Drawing for the job (mm, zero at the part's lowest x, y, z). A direction names the side the tool comes from. Round coordinates to 2 decimals unless told otherwise and drop trailing zeros. Loops run counter-clockwise (first coordinate to the right, second up) from the corner with the lowest first, then second, coordinate; pieces in that order, holes last. Notation, with made-up numbers: M 13.25,49.25 L 69.25,49.25 A16 ccw 69.25,71.25 Z; hole C 51,-3.75 d5. An arc over 180 degrees is marked long. Answer in a Markdown table with one row per item.
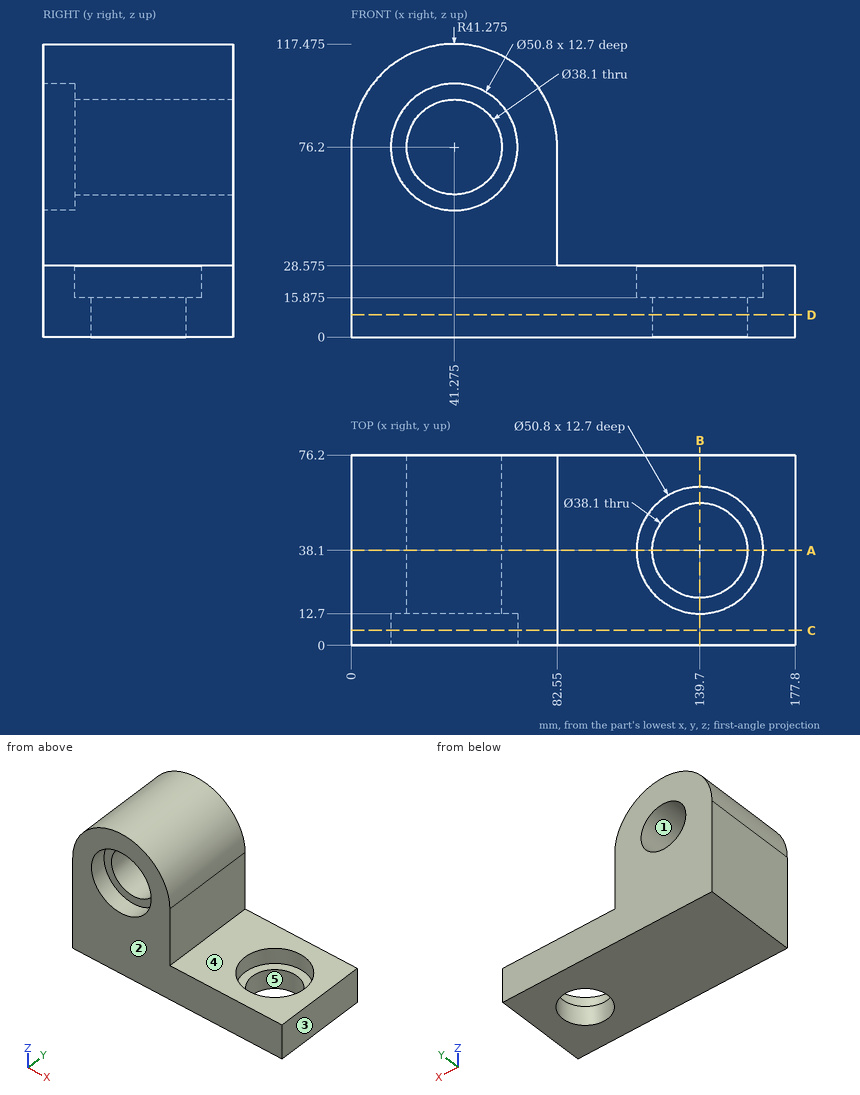
1. Saw through at A-A (y = 38.1). Write the cut outline in (x, z) (3 decimals), and give its area (3 significant figures).
Verdict:
| item | result |
|---|---|
| outline | M 0,0 L 120.65,0 L 120.65,15.875 L 114.3,15.875 L 114.3,28.575 L 82.55,28.575 L 82.55,76.2 A41.275 ccw 0,76.2 Z; M 158.75,0 L 177.8,0 L 177.8,28.575 L 165.1,28.575 L 165.1,15.875 L 158.75,15.875 Z; hole C 41.275,76.2 d38.1 |
| area | 9,300 mm² |
2. Saw through at B-B (x = 139.7). Write the cut outline in (y, z) (3 decimals).
Verdict:
| item | result |
|---|---|
| outline | M 0,0 L 19.05,0 L 19.05,15.875 L 12.7,15.875 L 12.7,28.575 L 0,28.575 Z; M 57.15,0 L 76.2,0 L 76.2,28.575 L 63.5,28.575 L 63.5,15.875 L 57.15,15.875 Z |
3. Saw through at D-D (z = 9). Write the cut outline in (x, y), and give its area (3 significant figures).
Verdict:
| item | result |
|---|---|
| outline | M 0,0 L 177.8,0 L 177.8,76.2 L 0,76.2 Z; hole C 139.7,38.1 d38.1 |
| area | 12,400 mm² |
4. Tool access for the marked faces 4 and 5: list every direction of +Z, -Z, +X, -X, +Y, -Y with a clear straight run to the whole face (end or side of a thin tool).
Verdict:
| item | result |
|---|---|
| face 4 | +Z, +X, +Y, -Y |
| face 5 | +Z, -Z |
5. Pin check, flat tips, straight feed: pin 1 (6 mm diameter, centred on y = 25, z = 71.5, fed in from +X); pin 2 (4 mm diameter, centred on x = 65, y = 10.5, fed in from +Z); pin 3 (6 mm diameter, centred on y = 56.5, z = 98.5, fed in from +X). Stop position of each tip, or through.
Verdict:
| item | result |
|---|---|
| pin 1 | stops at x = 82.55 |
| pin 2 | stops at z = 111.29 |
| pin 3 | stops at x = 77.76 |
6. Mould opens along X. For the marked faces 1, 2 and 3 say: +X half, -X half, draft (parallel to the pull), parting line (faces both ways), or undercut.
Verdict:
| item | result |
|---|---|
| face 1 | undercut |
| face 2 | draft |
| face 3 | +X half |
7. Saw through at C-C (y = 6). Write the cut outline in (x, z) (3 decimals), and give its area (3 significant figures).
Verdict:
| item | result |
|---|---|
| outline | M 0,0 L 177.8,0 L 177.8,28.575 L 82.55,28.575 L 82.55,76.2 A41.275 ccw 0,76.2 Z; hole C 41.275,76.2 d50.8 |
| area | 9,660 mm² |
8. Wall check: probe 1 along Y at (x, z) = (139.7, 8.5); probe 2 along Z at (x, y) = (40, 38); probe 3 along Z at (x, y) = (87, 52) (3 decimals). Give the ranges that are in metal, low to high.
Verdict:
| item | result |
|---|---|
| probe 1 | y = 0 to 19.05, 57.15 to 76.2 |
| probe 2 | z = 0 to 57.19, 95.21 to 117.46 |
| probe 3 | z = 0 to 28.575 |
